The drawing under review shows one solid part. Ordinate dimensions are in mm from its lowest x, y, z. A direction names the side the tool comes from. Round coordinates to 2 decimals unless told otherwise and drop trailing zeros. Write each loop counter-clockwise with the first axis right and the second up, starting at its lowest first coordinate (ties: lowest second). Pieces come first, ordered by that corner, then holes.
Item 1: Add section A-A (y = 38.1). Give the boundary of the cut face in (x, z) (3 decimals), plus the area to 3 significant figures.
Item 2: To check wall thickness, follow L1, parallel to Z at x = 72, y = 50.5; L2, parallel to Y at x = 38.5, z = 32.5; L3, parallel to Y at x = 38.1, z = 59 (3 decimals). State the ranges of each line that lie inside material, in increasing order.
Item 3: Add section D-D (z = 31). Give the boundary of the cut face in (x, y) (3 decimals), plus the area to 3 significant figures.
Item 4: Machinability: for the marked faces 1 and 2, which of the approach directions +Z, -Z, +X, -X, +Y, -Y give a long, thin tool a straight path to every point of the face, cutting with its end or side? Answer none if there is none.
Item 5: Draft analysis for pull direction Z (two halves, no side actions). For the marked faces 3, 4, 5 and 6, state which applies: +Z half, -Z half, draft (parallel to the pull), parting line (faces both ways), or undercut.
Item 6: Clearance check with flat-ended pins moving along their axes: pin 1 Ø5 at (x, y) = (64.5, 38) entering from +Z (1 decimal); pin 2 Ø3 at (y, z) = (20.5, 23) entering from +X; pin 3 Ø4 at (x, z) = (68, 37) entering from +Y. State where each tip first meets the part, or that it passes through.
Item 7: Add section C-C (z = 89). Give the boundary of the cut face in (x, y) (3 decimals), plus the area to 3 significant figures.
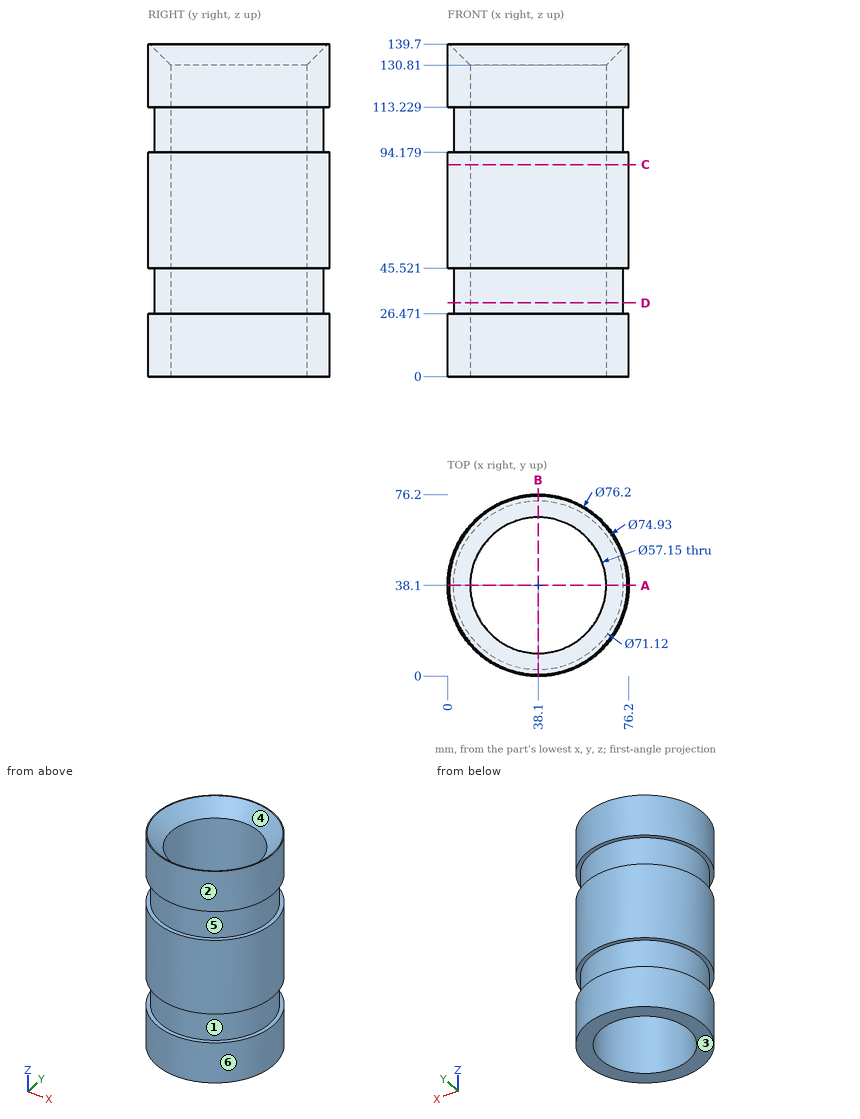
Numbers:
1. outline: (0, 0) - (9.525, 0) - (9.525, 130.81) - (0.635, 139.7) - (0, 139.7) - (0, 113.229) - (2.54, 113.229) - (2.54, 94.179) - (0, 94.179) - (0, 45.521) - (2.54, 45.521) - (2.54, 26.471) - (0, 26.471) - close; (66.675, 0) - (76.2, 0) - (76.2, 26.471) - (73.66, 26.471) - (73.66, 45.521) - (76.2, 45.521) - (76.2, 94.179) - (73.66, 94.179) - (73.66, 113.229) - (76.2, 113.229) - (76.2, 139.7) - (75.565, 139.7) - (66.675, 130.81) - close
1. area: 2,390 mm2
2. L1: z = 0 to 26.47, 45.52 to 94.18, 113.23 to 138.33
2. L2: y = 2.54 to 9.53, 66.67 to 73.66
2. L3: y = 0 to 9.525, 66.675 to 76.2
3. outline: circle Ø71.12 at (38.1, 38.1); hole circle Ø57.15 at (38.1, 38.1)
3. area: 1,410 mm2
4. face 1: none
4. face 2: +Z, -Z
5. face 3: -Z half
5. face 4: +Z half
5. face 5: undercut
5. face 6: draft
6. pin 1: stops at z = 131.1
6. pin 2: stops at x = 72.63
6. pin 3: stops at y = 60.15
7. outline: circle Ø76.2 at (38.1, 38.1); hole circle Ø57.15 at (38.1, 38.1)
7. area: 2,000 mm2
